Check sheet for the drawn part. Datum: minimum x, y, z corner. Units: mm. Coordinates: 2 decimals unless noted, no trailing zeros. Write each loop counter-clockwise with the first axis right and the second up, starting at its lowest first coordinate (ties: lowest second). Pieces come first, ordered by that corner, then holes. Notation, with made-up numbers: (-25.5, 7.5) -> (-10.5, 7.5) arc R21 cw to (-10.5, 39.5) -> close; hole circle Ø3 at (-8.75, 83). An arc over 180 degrees is marked (long way). Answer in a Markdown table with one row per item. Add a question column.
1. Depth check by flat-ended pin: P1, Ø1, axis at y = 2, z = 5.5, coming from the +X side; P2, Ø1, axis at y = 2.5, z = 21.5, coming from the +X side. Enter the tip coordinate at first touch or a pass-through.
2. Scan lines: L1, parallel to Y at x = 1.2, z = 13 (1 decimal); L2, parallel to X at y = 1.4, z = 32.5; L3, parallel to Y at x = 1.7, z = 34 (1 decimal). Record each from-to range of solid material in increasing order. Write a range as from..to.
3. Cross-section at A-A on z = 9. Record the cut outline in (x, y).
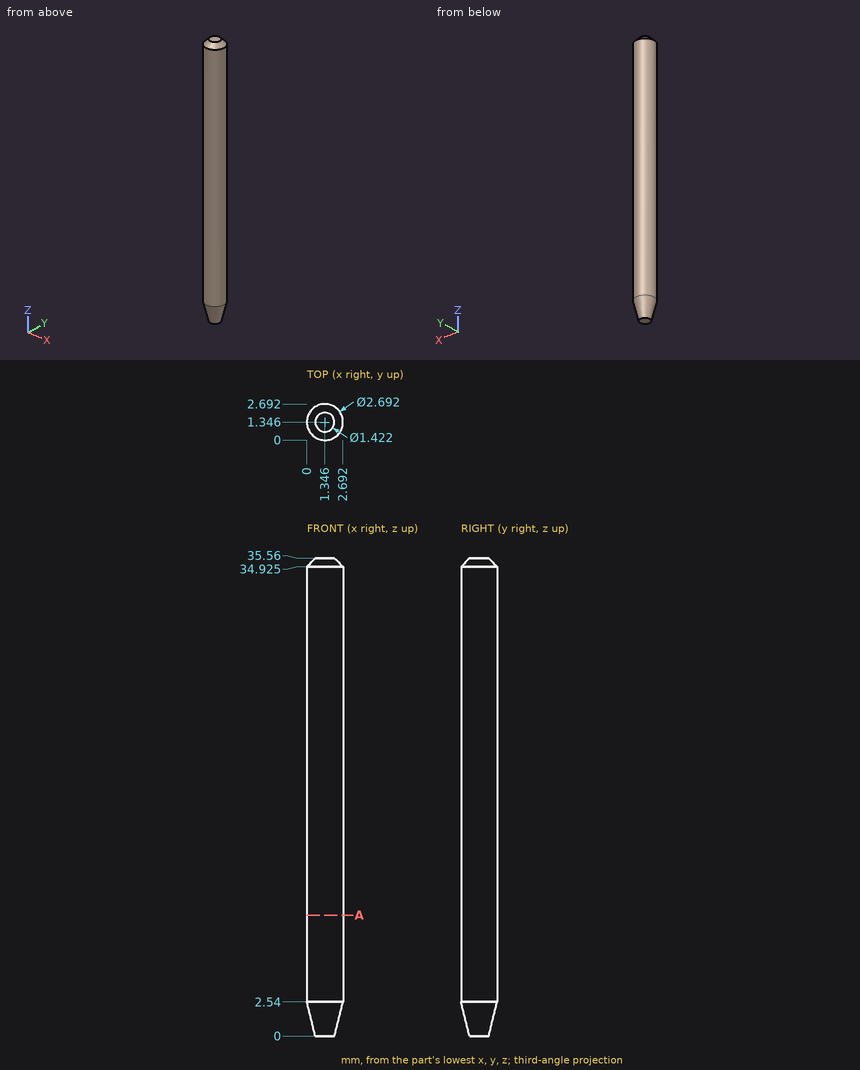
Results found:
| question | item | result |
|---|---|---|
| 1 | P1 | stops at x = 2.68 |
| 1 | P2 | stops at x = 2.52 |
| 2 | L1 | y = 0..2.7 |
| 2 | L2 | x = 0..2.69 |
| 2 | L3 | y = 0..2.6 |
| 3 | outline | circle Ø2.69 at (1.35, 1.35) |
